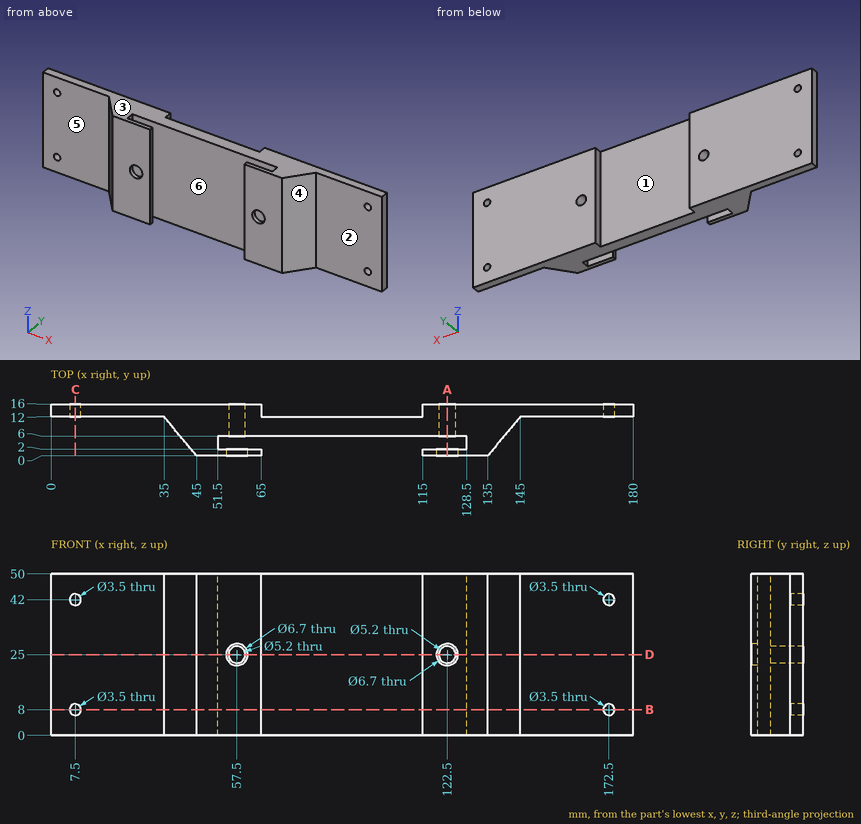
Geometry check sheet. Reference: drawing and pictorial views, mm from the part's lowest x, y, z. A direction names the side the tool comes from. Coordinates: 2 decimals unless noted, no trailing zeros. Order: outer loops, then holes, each group sorted by start corner. A loop starts at its lowest first (then second) coordinate and runs counter-clockwise, first axis right, second up.
1. Scan lines: line 1 (X direction, y = 15, z = 20); line 2 (Z direction, x = 7.5, y = 14.55); line 3 (Y direction, x = 125, z = 21). Record each from-to range of solid material in increasing order.
Results found:
line 1: x = 0 to 65, 115 to 180
line 2: z = 0 to 6.25, 9.75 to 40.25, 43.75 to 50
line 3: y = 0 to 2, 6 to 16
2. Release check for a two-part mould opening along X. For the marked faces 4, 5 and 6 record: +X half, -X half, draft (parallel to the pull), parting line (faces both ways), or undercut.
Results found:
face 4: +X half
face 5: draft
face 6: undercut
3. Sectioned sample at C-C, the plane x = 7.5. Record the cut outline in (y, z), and give its area (3 significant figures).
Results found:
outline: (12, 0) - (16, 0) - (16, 6.25) - (12, 6.25) - close; (12, 9.75) - (16, 9.75) - (16, 40.25) - (12, 40.25) - close; (12, 43.75) - (16, 43.75) - (16, 50) - (12, 50) - close
area: 172 mm2
4. Sectioned sample at B-B, the plane z = 8. Record the cut outline in (x, y), and give its area (3 significant figures).
Results found:
outline: (0, 12) - (5.75, 12) - (5.75, 16) - (0, 16) - close; (9.25, 12) - (35, 12) - (45, 0) - (65, 0) - (65, 2) - (51.5, 2) - (51.5, 6) - (128.5, 6) - (128.5, 2) - (115, 2) - (115, 0) - (135, 0) - (145, 12) - (170.75, 12) - (170.75, 16) - (115, 16) - (115, 12) - (65, 12) - (65, 16) - (9.25, 16) - close; (174.25, 12) - (180, 12) - (180, 16) - (174.25, 16) - close
area: 1,280 mm2
5. Set-up check for the marked faces 1, 2 and 3: record each of +Z, -Z, +X, -X, +Y, -Y from which the full face is reachable in a straight line by a thin tool's end or side.
Results found:
face 1: +Z, -Z, +Y
face 2: +Z, -Z, +X, -Y
face 3: +Z, +X, -X, +Y, -Y
6. Sectioned sample at D-D, the plane z = 25. Give the number of separate pieces and of enclosed holes in the cut face, and give its area (3 significant figures).
Results found:
separate pieces: 5
enclosed holes: 0
area: 1,180 mm2
7. Go/stop test with flat-tipped pins: pin 1 Ø5 at (y, z) = (3.5, 32.5) entering from +X; pin 2 Ø4.5 at (y, z) = (3.5, 23) entering from -X; pin 3 Ø5.5 at (x, z) = (57.5, 25) entering from -Y. Record where each tip stops, or that it passes through.
Results found:
pin 1: stops at x = 140
pin 2: stops at x = 40.21
pin 3: stops at y = 6
8. Sectioned sample at A-A, the plane x = 122.5. Record the cut outline in (y, z), and give its area (3 significant figures).
Results found:
outline: (0, 0) - (2, 0) - (2, 21.65) - (0, 21.65) - close; (0, 28.35) - (2, 28.35) - (2, 50) - (0, 50) - close; (6, 0) - (16, 0) - (16, 22.4) - (6, 22.4) - close; (6, 27.6) - (16, 27.6) - (16, 50) - (6, 50) - close
area: 535 mm2
